Answer from the drawing. Dimensions are ordinates in mm from the lowest x, y and z of the part. A direction names the side the tool comes from. Round coordinates to 2 decimals unless told otherwise and drop trailing zeros. Write each loop counter-clockwise with the first axis right and the second up, starting at its lowest first coordinate (ties: lowest second). Pieces come first, ordered by that corner, then holes. Notation, with made-up numbers: (-16, 7.5) -> (-1, 7.5) arc R34 cw to (-1, 38.5) -> close; hole circle Ø2 at (73.5, -6). An arc over 180 degrees is marked (long way). Return JSON: item names as keys, results as strings. Group by question number.
(1) A cutting plane is placed at C-C on z = 19. Give the vertices of the cut face in (x, y).
(2) A cutting plane is placed at D-D on x = 115.5. Give the vertices of the cut face in (y, z), then the cut area to 3 significant figures.
(3) Given pin 1 (2 mm diameter, centred on x = 102.5, z = 53.5, fed in from -Y); pin 2 (3 mm diameter, centred on x = 113, y = 6.5, fed in from +Z); pin 3 (2 mm diameter, centred on y = 3.5, z = 9.5, fed in from -X); pin 4 (5 mm diameter, centred on y = 1.5, z = 12.5, fed in from -X), each flat-ended and moving along its own axis, determine where each tip first touches the part or whether it passes through.
(4) Straight lines are drawn through the part: line 1 (X direction, y = 4.75, z = 30); line 2 (Z direction, x = 30, y = 2.25); line 3 (Z direction, x = 143, y = 9). For each, find the intervals that lie inside material, in ascending order.
(5) For the marked faces 1 and 2, determine the directions among +Z, -Z, +X, -X, +Y, -Y from which every point of the face is accessible in a straight line to the end or side of a thin tool.
(6) A cutting plane is placed at A-A on x = 30. Give the vertices of the cut face in (y, z), then the cut area to 3 significant figures.
(7) A cutting plane is placed at B-B on y = 2.5. Give the vertices of the cut face in (x, z).
(8) The mould has two halves that part along X. Classify the marked faces 3, 4 and 5: released by +X, released by -X, zero draft, split by the parting line, or undercut.
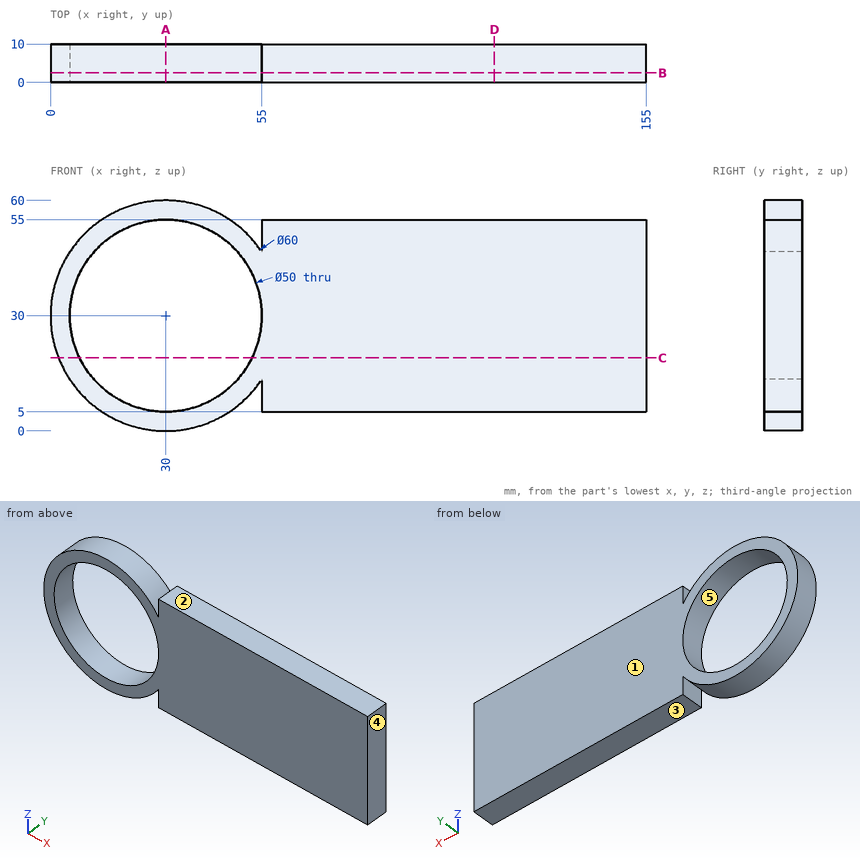
Checks:
{
 "1": {"outline": "(2.09, 0) -> (7.55, 0) -> (7.55, 10) -> (2.09, 10) -> close; (52.45, 0) -> (155, 0) -> (155, 10) -> (52.45, 10) -> close"},
 "2": {"outline": "(0, 5) -> (10, 5) -> (10, 55) -> (0, 55) -> close", "area": "500 mm^2"},
 "3": {"pin 1": "stops at y = 0", "pin 2": "stops at z = 55", "pin 3": "stops at x = 7.2", "pin 4": "stops at x = 4.02"},
 "4": {"line 1": "x = 0 to 5, 55 to 155", "line 2": "z = 0 to 5, 55 to 60", "line 3": "z = 5 to 55"},
 "5": {"face 1": "+Z, -Z, +X, -X, +Y", "face 2": "+Z, +X, +Y, -Y"},
 "6": {"outline": "(0, 0) -> (10, 0) -> (10, 5) -> (0, 5) -> close; (0, 55) -> (10, 55) -> (10, 60) -> (0, 60) -> close", "area": "100 mm^2"},
 "7": {"outline": "(55, 5) -> (155, 5) -> (155, 55) -> (55, 55) -> (55, 46.58) arc R30 ccw (long way) to (55, 13.42) -> close; hole circle Ø50 at (30, 30)"},
 "8": {"face 3": "zero draft", "face 4": "released by +X", "face 5": "undercut"}
}
